```python
from build123d import *

# Parameters (mm, degrees)
F1_DEPTH = 20
F2_SIZE  = 1
F3_R     = 2.5
F4_DEPTH = 25
F6_DEPTH = 6


with BuildPart() as f1:
    # F0 (on Front) → F1 (new body)
    with BuildSketch(Plane.XZ):
        Polygon((-44.529999, 7.5), (-44.529999, -17.5), (-39.529999, -17.5), (-39.529999, 2.5), (-19.529999, 2.5), (-19.529999, -7.5), (0, -7.5), (46.96333, -7.5), (46.96333, 0), (28.470001, 0), (28.470001, 7.5), (0, 7.5), align=None)
    extrude(amount=F1_DEPTH)

    # F2
    f2_edges = [f1.edges().sort_by_distance(p)[0] for p in [
        (-8.029999, -20, 7.5),
        (-8.029999, 0, 7.5),
        (-44.529999, -10, 7.5),
        (-44.529999, -20, -5),
        (-44.529999, 0, -5),
        (-44.529999, -10, -17.5),
        (13.716665, 0, -7.5),
        (13.716665, -20, -7.5),
    ]]
    chamfer(f2_edges, length=F2_SIZE)

    # F3 (on face) → F4 (cut)
    with BuildSketch(Plane(origin=(0, 0, -7.5), x_dir=(1, 0, 0), z_dir=(0, 0, -1))):
        with Locations((-29.529999, 10)):
            Circle(F3_R)
        with Locations((39.46333, 10)):
            Circle(F3_R)
    extrude(amount=-F4_DEPTH, mode=Mode.SUBTRACT)

    # F5 (on face) → F6 (cut)
    with BuildSketch(Plane(origin=(0, 0, -7.5), x_dir=(1, 0, 0), z_dir=(0, 0, -1))):
        Polygon((35.133203, 12.5), (35.133203, 7.5), (39.46333, 5), (43.793457, 7.5), (43.793457, 12.5), (39.46333, 15), align=None)
    extrude(amount=-F6_DEPTH, mode=Mode.SUBTRACT)


solid = f1.part
```
Build history of the part. All positions in model axes, mm. A direction names the side the tool comes from. Give positions to 0.01 mm unless a question says otherwise; leave off trailing zeros. Loops run counter-clockwise (first coordinate to the right, second up) from the corner with the lowest first, then second, coordinate; pieces in that order, holes last. Notation, with made-up numbers: (48, 15) -> (55, 15) arc R16 ccw to (55, 35) -> close; hole circle Ø10 at (-23.75, 13). An arc over 180 degrees is marked (long way). One line per question, with ' | ' between items.
Q1. Cut at A-A, the plane z = -3.25. Write the cut outline in (x, y).
Filled sheet:
outline: (-44.53, -19) -> (-43.53, -20) -> (-39.53, -20) -> (-39.53, 0) -> (-43.53, 0) -> (-44.53, -1) -> close; (-19.53, -20) -> (46.96, -20) -> (46.96, 0) -> (-19.53, 0) -> close; hole (35.13, -12.5) -> (39.46, -15) -> (43.79, -12.5) -> (43.79, -7.5) -> (39.46, -5) -> (35.13, -7.5) -> close
Q2. Drill centre lines: line 1 along X through (y, z) = (-10, -0.5); line 2 along X through (y, z) = (-14, -0.5); line 3 along X through (y, z) = (-10, 5.7). Where is each one in solid material? Low to high. Write a range as [from, to].
Filled sheet:
line 1: x = [-44.53, -39.53], [-19.53, 36.96], [41.96, 46.96] | line 2: x = [-44.53, -39.53], [-19.53, 46.96] | line 3: x = [-44.53, -32.03], [-27.03, 28.47]
Q3. Tool access for faces 5 (the flat face through (-39.53, -10, -8)), 6 (the flat face through (36, -10, 0)), 7 (the flat face through (-42, -10, -17.5)), 8 (the flat face through (43.793, -10, -5)): list every direction of +Z, -Z, +X, -X, +Y, -Y with a clear straight run to the whole face (end or side of a thin tool).
Filled sheet:
face 5: -Z, +Y, -Y | face 6: +Z, +X, +Y, -Y | face 7: -Z, +X, -X, +Y, -Y | face 8: -Z
Q4. Cut at D-D, the plane z = -12. Write the cut outline in (x, y).
Filled sheet:
outline: (-44.53, -19) -> (-43.53, -20) -> (-39.53, -20) -> (-39.53, 0) -> (-43.53, 0) -> (-44.53, -1) -> close
Q5. Pull direction X, two halves, no side cores. Call faces 1 (the flat face through (41.66, -13.73, -4.54)), 2 (the flat face through (37.268, -6.268, -4.542)), 3 (the flat face through (46.963, -10, -4)), 4 (the flat face through (13, -10, -7.5)): pulls with the +X half, pulls with the -X half, needs draft (parallel to the pull), parting line crosses it, or undercut.
Filled sheet:
face 1: undercut | face 2: undercut | face 3: pulls with the +X half | face 4: needs draft
Q6. Cut at C-C, the plane x = -8.5. Write the cut outline in (y, z).
Filled sheet:
outline: (-20, -6.5) -> (-19, -7.5) -> (-1, -7.5) -> (0, -6.5) -> (0, 6.5) -> (-1, 7.5) -> (-19, 7.5) -> (-20, 6.5) -> close
Q7. Drop flat-ended pins along their axis: pin 1 (7 mm diameter, centred on x = 39, y = -11.5, fed in from -Z); pin 2 (9 mm diameter, centred on x = 34, y = -9, fed in from +Z); pin 3 (4.5 mm diameter, centred on x = -29.53, y = -10, fed in from +Z); pin 4 (8 mm diameter, centred on y = -10, z = 4.5, fed in from +X). Give the stop position or say it passes through.
Filled sheet:
pin 1: stops at z = -7.5 | pin 2: stops at z = 0 | pin 3: passes through | pin 4: stops at x = 28.47
Q8. Cut at B-B, the plane y = -10. Write the cut outline in (x, z).
Filled sheet:
outline: (-44.53, -16.5) -> (-43.53, -17.5) -> (-39.53, -17.5) -> (-39.53, 2.5) -> (-32.03, 2.5) -> (-32.03, 7.5) -> (-43.53, 7.5) -> (-44.53, 6.5) -> close; (-27.03, 2.5) -> (-19.53, 2.5) -> (-19.53, -7.5) -> (35.13, -7.5) -> (35.13, -1.5) -> (36.96, -1.5) -> (36.96, 0) -> (28.47, 0) -> (28.47, 7.5) -> (-27.03, 7.5) -> close; (41.96, -1.5) -> (43.79, -1.5) -> (43.79, -7.5) -> (46.96, -7.5) -> (46.96, 0) -> (41.96, 0) -> close
